from build123d import *

# Parameters (mm, degrees)
F0_W     = 8.2
F0_H     = 8.2
F1_DEPTH = 10
F2_R     = 9.25
F3_DEPTH = 5.5


with BuildPart() as f1:
    # F0 (on Top) → F1 (new body)
    with BuildSketch(Plane.XY):
        with BuildLine():
            ThreePointArc((15, 5.5), (14.414214, 6.914214), (13, 7.5))
            Line((13, 7.5), (-13, 7.5))
            ThreePointArc((-13, 7.5), (-14.414214, 6.914214), (-15, 5.5))
            Line((-15, 5.5), (-15, -5.5))
            ThreePointArc((-15, -5.5), (-14.414214, -6.914214), (-13, -7.5))
            Line((-13, -7.5), (13, -7.5))
            ThreePointArc((13, -7.5), (14.414214, -6.914214), (15, -5.5))
            Line((15, -5.5), (15, 5.5))
        make_face()
        Rectangle(F0_W, F0_H, mode=Mode.SUBTRACT)
    extrude(amount=F1_DEPTH)

    # F2 (on face) → F3 (cut)
    with BuildSketch(Plane.XY.offset(10)):
        Circle(F2_R)
    extrude(amount=-F3_DEPTH, mode=Mode.SUBTRACT)


solid = f1.part
Geometry: final body of the model. Coordinates: model frame, mm. A direction names the side the tool comes from. Round coordinates to 2 decimals unless told otherwise and drop trailing zeros. Order: outer loops, then holes, each group sorted by start corner. A loop starts at its lowest first (then second) coordinate and runs counter-clockwise, first axis right, second up.
Q1. Pin query (flat end, axial travel): pin 1 (7.5 mm diameter, centred on x = -0.5, y = -0.5, fed in from +Z). Return the tip coordinate at first contact, or that it passes through.
Result sheet:
pin 1: stops at z = 4.5
Q2. Access query for faces 5 (the face through (0, -5, 4.5)), 6 (the face through (0, 5, 0)), 7 (the face through (-4.1, 0, 2)). Directions: +Z, -Z, +X, -X, +Y, -Y. A direction counts if a zero-diameter tool reaches every point of the face in a straight line with its end or side. Return the directions, or none.
Result sheet:
face 5: +Z
face 6: -Z, +X, -X, +Y, -Y
face 7: +Z, -Z
Q3. Material intervals for probe 1 along X at (y, z) = (0.5, 4.25); probe 2 along Y at (x, z) = (-4, 1.5); probe 3 along X at (y, z) = (-1.25, 5), sorted ascending.
Result sheet:
probe 1: x = -15 to -4.1, 4.1 to 15
probe 2: y = -7.5 to -4.1, 4.1 to 7.5
probe 3: x = -15 to -9.17, 9.17 to 15
Q4. Section D-D, the plane y = -1.25. Output: boundary loops of the cut face in (x, z).
Result sheet:
outline: (-15, 0) - (-4.1, 0) - (-4.1, 4.5) - (-9.17, 4.5) - (-9.17, 10) - (-15, 10) - close; (4.1, 0) - (15, 0) - (15, 10) - (9.17, 10) - (9.17, 4.5) - (4.1, 4.5) - close
Q5. Section C-C, the plane z = 8.75. Output: boundary loops of the cut face in (x, y), and give its area (3 significant figures).
Result sheet:
outline: (-15, -5.5) arc R2 ccw to (-13, -7.5) - (-5.41, -7.5) arc R9.25 cw to (-5.41, 7.5) - (-13, 7.5) arc R2 ccw to (-15, 5.5) - close; (5.41, -7.5) - (13, -7.5) arc R2 ccw to (15, -5.5) - (15, 5.5) arc R2 ccw to (13, 7.5) - (5.41, 7.5) arc R9.25 cw to start
area: 204 mm2
Q6. Section B-B, the plane z = 0.5. Output: boundary loops of the cut face in (x, y), and give its area (3 significant figures).
Result sheet:
outline: (-15, -5.5) arc R2 ccw to (-13, -7.5) - (13, -7.5) arc R2 ccw to (15, -5.5) - (15, 5.5) arc R2 ccw to (13, 7.5) - (-13, 7.5) arc R2 ccw to (-15, 5.5) - close; hole (-4.1, -4.1) - (4.1, -4.1) - (4.1, 4.1) - (-4.1, 4.1) - close
area: 379 mm2
Q7. Section A-A, the plane x = 1. Output: boundary loops of the cut face in (y, z), and give its area (3 significant figures).
Result sheet:
outline: (-7.5, 0) - (-4.1, 0) - (-4.1, 4.5) - (-7.5, 4.5) - close; (4.1, 0) - (7.5, 0) - (7.5, 4.5) - (4.1, 4.5) - close
area: 30.6 mm2
Q8. Mould query, pull axis Y, two halves, no side actions, for faces 1 (the face through (0, -4.1, 2)), 2 (the face through (14.43, 6.9, 4.93)), 3 (the face through (-9.25, 0.12, 7.29)), 4 (the face through (15, 0, 5)). Classes: released by +Y, released by -Y, zero draft, split by the parting line, or undercut.
Result sheet:
face 1: undercut
face 2: released by +Y
face 3: undercut
face 4: zero draft
